Job drawing, mm, ordinate dimensions from the low corner. One solid piece. A direction names the side the tool comes from. Give positions to 0.01 mm unless a question says otherwise; leave off trailing zeros. Write each loop counter-clockwise with the first axis right and the second up, starting at its lowest first coordinate (ties: lowest second). Pieces come first, ordered by that corner, then holes. Notation, with made-up numbers: (46.25, 64.25) - (83.25, 64.25) arc R19 ccw to (83.25, 92.25) - close; hole circle Ø11 at (72.25, -6). An arc over 180 degrees is marked (long way). Answer as a JSON object with one key per item and string values.
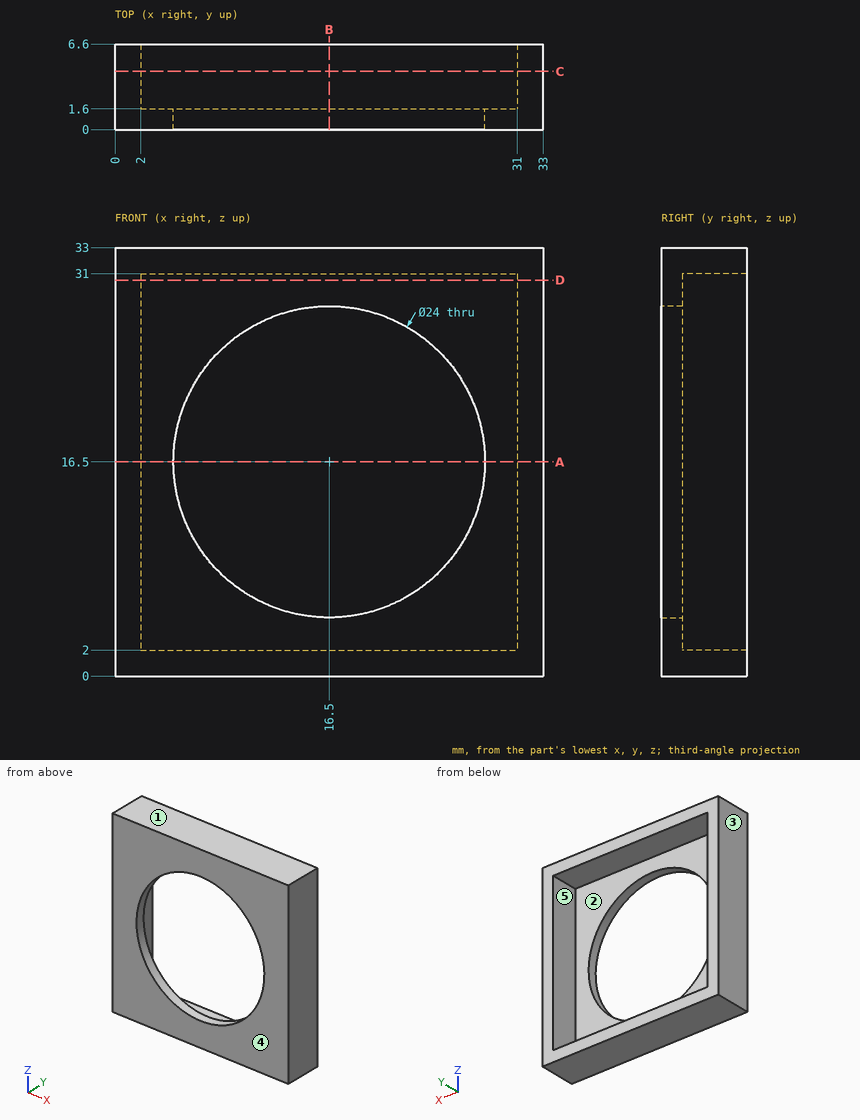
Item 1: Cut at B-B (x = 16.5). Give the cut face in (y, z), and give its area (3 significant figures).
Entries:
{"outline": "(0, 0) - (6.6, 0) - (6.6, 2) - (1.6, 2) - (1.6, 4.5) - (0, 4.5) - close; (0, 28.5) - (1.6, 28.5) - (1.6, 31) - (6.6, 31) - (6.6, 33) - (0, 33) - close", "area": "34.4 mm2"}
Item 2: Cut at D-D (z = 30.5). Give the cut face in (x, y), and give its area (3 significant figures).
Entries:
{"outline": "(0, 0) - (33, 0) - (33, 6.6) - (31, 6.6) - (31, 1.6) - (2, 1.6) - (2, 6.6) - (0, 6.6) - close", "area": "72.8 mm2"}
Item 3: Cut at A-A (z = 16.5). Give the cut face in (x, y).
Entries:
{"outline": "(0, 0) - (4.5, 0) - (4.5, 1.6) - (2, 1.6) - (2, 6.6) - (0, 6.6) - close; (28.5, 0) - (33, 0) - (33, 6.6) - (31, 6.6) - (31, 1.6) - (28.5, 1.6) - close"}
Item 4: Mould opens along Z. For the marked faces 1, 2 and 3 say: +Z half, -Z half, draft (parallel to the pull), parting line (faces both ways), or undercut.
Entries:
{"face 1": "+Z half", "face 2": "undercut", "face 3": "draft"}
Item 5: Which spindle directions (+Z, -Z, +X, -X, +Y, -Y) get a long thin tool onto all of the face, cutting with end or side? Do the marked faces 4 and 5. Say none if no direction does.
Entries:
{"face 4": "+Z, -Z, +X, -X, -Y", "face 5": "+Y"}
Item 6: Probe line 1 (X direction, y = 1.15, z = 16.5); line 2 (X direction, y = 5.75, z = 10). List the from-to ranges inside material, lowest first. Write a range as from..to.
Entries:
{"line 1": "0..4.5, 28.5..33", "line 2": "0..2, 31..33"}
Item 7: Cut at C-C (y = 4.5). Give the cut face in (x, z).
Entries:
{"outline": "(0, 0) - (33, 0) - (33, 33) - (0, 33) - close; hole (2, 2) - (31, 2) - (31, 31) - (2, 31) - close"}
Item 8: Flat gauge pin, fed straight in: P1, Ø1.5, axis at y = 1, z = 19, coming from the -X side. Where does the tip first touch, or does it go through?
Entries:
{"P1": "x = 0"}
